from build123d import *

# Parameters (mm, degrees)
SKETCH1_R           = 40
BOSS_EXTRUDE1_DEPTH = 21
FILLET1_R           = 10
FILLET2_R           = 10
FILLET3_R           = 10
FILLET4_R           = 10
FILLET5_R           = 5
FILLET6_R           = 5
FILLET7_R           = 75
FILLET8_R           = 75
SKETCH2_R           = 3
CUT_EXTRUDE1_DEPTH  = 164.836129338


with BuildPart() as part:
    # Sketch1 → Boss-Extrude1 (new body)
    with BuildSketch(Plane(origin=(0, 0, 0), x_dir=(1, 0, 0), z_dir=(0, 1, 0))):
        Polygon((0.191150297, -52.534941872), (103.191150297, -52.534941872), (103.191150297, -40), (72.191150297, -40), (72.191150297, 85), (0.191150297, 85), (-72.808849703, 85), (-72.808849703, -40), (-103.808849703, -40), (-103.808849703, -52.534941872), align=None)
        with Locations(Location((-0.308849703, 12.94638448, 0), (0, 0, 90))):
            Circle(SKETCH1_R, mode=Mode.SUBTRACT)
    extrude(amount=BOSS_EXTRUDE1_DEPTH)

    # Fillet1
    fillet1_edges = [part.edges().sort_by_distance(p)[0] for p in [
        (103.191150297, 21, 46.267470936),
    ]]
    fillet(fillet1_edges, radius=FILLET1_R)

    # Fillet2
    fillet2_edges = [part.edges().sort_by_distance(p)[0] for p in [
        (-103.808849703, 21, 46.267470936),
    ]]
    fillet(fillet2_edges, radius=FILLET2_R)

    # Fillet3
    fillet3_edges = [part.edges().sort_by_distance(p)[0] for p in [
        (-103.808849703, 0, 46.267470936),
    ]]
    fillet(fillet3_edges, radius=FILLET3_R)

    # Fillet4
    fillet4_edges = [part.edges().sort_by_distance(p)[0] for p in [
        (103.191150297, 0, 46.267470936),
    ]]
    fillet(fillet4_edges, radius=FILLET4_R)

    # Fillet5
    fillet5_edges = [part.edges().sort_by_distance(p)[0] for p in [
        (72.191150297, 10.5, 40),
    ]]
    fillet(fillet5_edges, radius=FILLET5_R)

    # Fillet6
    fillet6_edges = [part.edges().sort_by_distance(p)[0] for p in [
        (-72.808849703, 10.5, 40),
    ]]
    fillet(fillet6_edges, radius=FILLET6_R)

    # Fillet7
    fillet7_edges = [part.edges().sort_by_distance(p)[0] for p in [
        (-72.808849703, 10.5, -85),
    ]]
    fillet(fillet7_edges, radius=FILLET7_R)

    # Fillet8
    # the kernel refuses this fillet: 75 mm, written as the material it takes off along each edge
    with BuildSketch(Plane(origin=(72.191150297, -187.082869339, -85), x_dir=(-1, 0, 0), z_dir=(0, 1, 0))) as fillet8_piece_1:
        with BuildLine():
            CenterArc((75, 74.833147735), FILLET8_R, 180, 86.177446271)
            Line((0, 74.833147735), (-1.5, 74.833147735))
            Line((-1.5, 74.833147735), (-1.5, 0))
            Line((-1.5, 0), (0, -1.5))
            ThreePointArc((0, -1.5), (35, -1.5), (69.9, -1.496662955))
            Line((69.9, -1.496662955), (70, 0))
        make_face()
    extrude(amount=395.165738677, mode=Mode.SUBTRACT)

    # Sketch2 → Cut-Extrude1 (cut, through all)
    with BuildSketch(Plane(origin=(0, 0, 40), x_dir=(-1, 0, 0), z_dir=(0, 0, -1))):
        with Locations((-90.191150297, 10.5)):
            Circle(SKETCH2_R)
        with Locations(Location((90.191150297, 10.5, 0), (0, 0, 180))):
            Circle(SKETCH2_R)
    extrude(amount=-CUT_EXTRUDE1_DEPTH, mode=Mode.SUBTRACT)


solid = part.part
Source: CAD feature listing. Evaluate the final solid. Frame: model axes, mm. A direction names the side the tool comes from. Round coordinates to 2 decimals unless told otherwise and drop trailing zeros. Write each loop counter-clockwise with the first axis right and the second up, starting at its lowest first coordinate (ties: lowest second). Pieces come first, ordered by that corner, then holes. Notation, with made-up numbers: M 10,63.25 L 66,63.25 A10 cw 66,72.25 Z; hole C 2.25,17.25 d1. An arc over 180 degrees is marked long. One line per item, written item: value. Start each with the question number.
Item 1: Section query A-A (x = -13.5). Return the cut outline in (y, z).
Item 2: Pin query (flat end, axial travel): pin 1 (1.5 mm diameter, centred on x = -48, y = 16, fed in from -Z); pin 2 (1 mm diameter, centred on x = 81, y = 14, fed in from -Z); pin 3 (10.5 mm diameter, centred on y = 13, z = 15, fed in from -X). Return the tip coordinate at first contact, or that it passes through.
Item 3: Section query B-B (y = 17). Return the cut outline in (x, z).
Item 4: Set-up query: faces 5 (the flat face through (87, 8, 40)), 6 (the flat face through (-88, 8, 40)), 7 (the cylindrical face through (87.33, 11.4, 46.18)). Return all of +Z, -Z, +X, -X, +Y, -Y with unobstructed straight access to the full face (end or side cutting, diameter ignored); none if empty.
Item 5: Mould query, pull axis Y, two halves, no side actions, for faces 1 (the cylindrical face through (-100.96, 3.01, 46.36)), 2 (the cylindrical face through (-87.33, 9.6, 46.18)), 3 (the flat face through (-2, 10, 52.535)), 4 (the cylindrical face through (100.34, 17.99, 46.18)). Classes: pulls with the +Y half, pulls with the -Y half, needs draft (parallel to the pull), parting line crosses it, or undercut.
Item 6: Ray query, L1, parallel to Y at x = 90.5, z = 43; L2, parallel to Z at x = 93, y = 5.75; L3, parallel to Z at x = -5.5, y = 4.25. Return the intervals inside material, ascending. Write a range as from..to.
Item 7: Section query C-C (z = -21). Return the cut outline in (x, y), plus the area to 3 significant figures.
Item 8: Section query D-D (y = 3.5). Return the cut outline in (x, z), plus the area to 3 significant figures.
Result set:
1. outline: M 0,-83.34 L 21,-83.34 L 21,-50.71 L 0,-50.71 Z; M 0,24.82 L 21,24.82 L 21,52.53 L 0,52.53 Z
2. pin 1: stops at z = -66.4
2. pin 2: stops at z = 40
2. pin 3: stops at x = -72.81
3. outline: M -101.81,40 L -77.81,40 A5 cw -72.81,35 L -72.81,-10 A75 ccw 2.19,-85 A75 ccw 72.19,-10.17 L 72.19,35 A5 cw 77.19,40 L 101.19,40 L 101.19,52.53 L -101.81,52.53 Z; hole C -0.31,-12.95 d80
4. face 5: -Z, +X, +Y, -Y
4. face 6: -Z, -X, +Y, -Y
4. face 7: +Z, -Z
5. face 1: pulls with the -Y half
5. face 2: undercut
5. face 3: needs draft
5. face 4: pulls with the +Y half
6. L1: y = 0..7.52, 13.48..21
6. L2: z = 40..52.53
6. L3: z = -84.6..-52.61, 26.72..52.53
7. outline: M -72,0 L -39.49,0 L -39.49,21 L -72,21 Z; M 38.87,0 L 71.4,0 L 71.4,21 L 38.87,21 Z
7. area: 1,370 mm²
8. outline: M -101.41,40 L -77.81,40 A5 cw -72.81,35 L -72.81,-10 A75 ccw 2.19,-85 A75 ccw 72.19,-10.17 L 72.19,35 A5 cw 77.19,40 L 100.79,40 L 100.79,52.53 L -101.41,52.53 Z; hole C -0.31,-12.95 d80
8. area: 13,200 mm²
